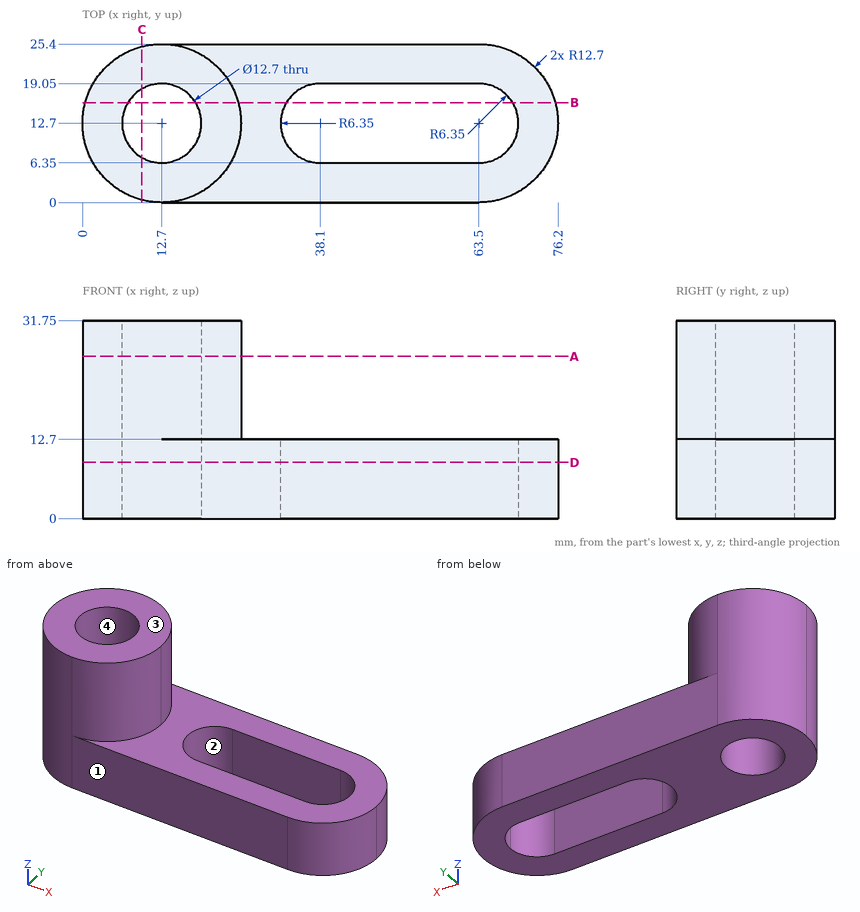
Here's the drawing with two shaded views (mm, measured from the low corner). I have some questions. A direction names the side the tool comes from. Coordinates: 2 decimals unless noted, no trailing zeros. Write each loop counter-clockwise with the first axis right and the second up, starting at its lowest first coordinate (ties: lowest second). Pieces come first, ordered by that corner, then holes. Notation, with made-up numbers: M 17.25,73 L 23.25,73 A25 cw 23.25,101 Z; hole C 8,36 d2. An arc over 180 degrees is marked long. Answer as CSV lines item,"result".
Item 1: We'd pull the mould along X, two halves only. Please class the marked faces 3 and 4: +X half, -X half, draft (parallel to the pull), parting line (faces both ways), or undercut.
Geometry results:
face 3,"draft"
face 4,"undercut"
Item 2: Imagine slicing it at B-B on y = 16. List the corners of the cut face in (x, z) for me, plus the area to 3 significant figures.
Geometry results:
outline,"M 0.44,0 L 7.27,0 L 7.27,31.75 L 0.44,31.75 Z; M 18.13,0 L 32.67,0 L 32.67,12.7 L 24.96,12.7 L 24.96,31.75 L 18.13,31.75 Z; M 68.93,0 L 75.76,0 L 75.76,12.7 L 68.93,12.7 Z"
area,"619 mm2"
Item 3: Imagine slicing it at A-A on z = 26. List the corners of the cut face in (x, y) for me.
Geometry results:
outline,"C 12.7,12.7 d25.4; hole C 12.7,12.7 d12.7"
Item 4: I'm going to push flat-ended pins straight in: P1, Ø8, axis at y = 12, z = 4, coming from the -X side; P2, Ø4, axis at y = 13, z = 24, coming from the +X side; P3, Ø2, axis at y = 22, z = 16.5, coming from the -X side; P4, Ø10, axis at y = 7, z = 8.5, coming from the +X side. Where does each tip first touch, or does it pass through?
Geometry results:
P1,"stops at x = 0"
P2,"stops at x = 25.4"
P3,"stops at x = 3.09"
P4,"stops at x = 76.18"
Item 5: Imagine slicing it at C-C on x = 9.5. List the corners of the cut face in (y, z) for me, plus the area to 3 significant figures.
Geometry results:
outline,"M 0.41,0 L 7.22,0 L 7.22,31.75 L 0.41,31.75 Z; M 18.18,0 L 24.99,0 L 24.99,31.75 L 18.18,31.75 Z"
area,"432 mm2"
Item 6: Imagine slicing it at D-D on z = 9. List the corners of the cut face in (x, y) for me, plus the area to 3 significant figures.
Geometry results:
outline,"M 12.7,0 L 63.5,0 A12.7 ccw 63.5,25.4 L 12.7,25.4 A12.7 ccw Z; hole C 12.7,12.7 d12.7; hole M 38.1,6.35 L 63.5,6.35 A6.35 ccw 63.5,19.05 L 38.1,19.05 A6.35 ccw Z"
area,"1,220 mm2"
Item 7: On a 3-axis mill with a long thin cutter (end or side, diameter ignored), from which of +Z, -Z, +X, -X, +Y, -Y can I reach the whole of each face in a straight line? I mean the marked faces 1 and 2. Say none if no direction works.
Geometry results:
face 1,"+Z, -Z, +X, -X, -Y"
face 2,"+Z, -Z"
Item 8: Please list where these lines run through material, in increasing order: line 1 along X through (y, z) = (10.25, 2.5); line 2 along Z through (x, y) = (71, 11.5); line 3 along X through (y, z) = (17.5, 18.5).
Geometry results:
line 1,"x = 0.24 to 6.84, 18.56 to 32.24, 69.36 to 75.96"
line 2,"z = 0 to 12.7"
line 3,"x = 0.94 to 8.54, 16.86 to 24.46"
